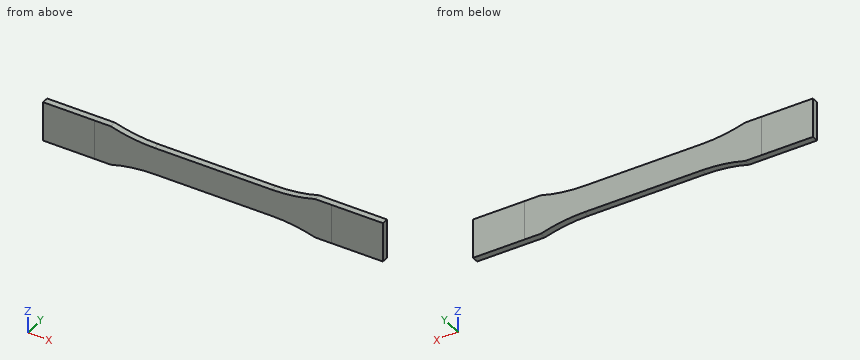
```python
from build123d import *

# Parameters (mm, degrees)
CROQUIS1_W              = 57
CROQUIS1_H              = 13
SALIENTE_EXTRUIR1_DEPTH = 1.6
CROQUIS2_W              = 25
CROQUIS2_H              = 19
CORTAR_EXTRUIR1_DEPTH   = 0.01


with BuildPart() as part:
    # Croquis1 → Saliente-Extruir1 (new body, symmetric)
    with BuildSketch(Plane(origin=(0, 0, 0), x_dir=(1, 0, 0), z_dir=(0, 1, 0))):
        with BuildLine():
            Line((-82.5, -9.5), (-49.642374512, -9.5))
            ThreePointArc((-49.642374512, -9.5), (-39.177078252, -7.253737634), (-28.5, -6.5))
            Line((-28.5, -6.5), (-28.5, 6.5))
            ThreePointArc((-28.5, 6.5), (-39.177078252, 7.253737634), (-49.642374512, 9.5))
            Line((-49.642374512, 9.5), (-82.5, 9.5))
            Line((-82.5, 9.5), (-82.5, -9.5))
        make_face()
        with BuildLine():
            Line((49.642374512, -9.5), (82.5, -9.5))
            Line((82.5, -9.5), (82.5, 9.5))
            Line((82.5, 9.5), (49.642374512, 9.5))
            ThreePointArc((49.642374512, 9.5), (39.177078252, 7.253737634), (28.5, 6.5))
            Line((28.5, 6.5), (28.5, -6.5))
            ThreePointArc((28.5, -6.5), (39.177078252, -7.253737634), (49.642374512, -9.5))
        make_face()
        Rectangle(CROQUIS1_W, CROQUIS1_H)
    extrude(amount=SALIENTE_EXTRUIR1_DEPTH, both=True)

    # Croquis2 → Cortar-Extruir1 (cut)
    with BuildSketch(Plane(origin=(0, 1.6, 0), x_dir=(1, 0, 0), z_dir=(0, 1, 0))):
        with Locations((-70, 0)):
            Rectangle(CROQUIS2_W, CROQUIS2_H)
        with Locations((70, 0)):
            Rectangle(CROQUIS2_W, CROQUIS2_H)
    cortar_extruir1 = extrude(amount=-CORTAR_EXTRUIR1_DEPTH, mode=Mode.SUBTRACT)

    # Simetría1: Cortar-Extruir1 across plane
    add(cortar_extruir1.mirror(Plane.ZX), mode=Mode.SUBTRACT)


solid = part.part
```
Source: CAD feature listing. Evaluate the final solid. Frame: model axes, mm. Round coordinates to 2 decimals unless told otherwise and drop trailing zeros. Loops run counter-clockwise (first coordinate to the right, second up) from the corner with the lowest first, then second, coordinate; pieces in that order, holes last.
1. Section query A-A on y = 0.75. Output: boundary loops of the cut face in (x, z), and give its area (3 significant figures).
2. Section query B-B on x = -1. Output: boundary loops of the cut face in (y, z), and give its area (3 significant figures).
3. Ray query, L1, parallel to Y at x = -69.5, z = 2.5; L2, parallel to Z at x = -2, y = -0.75; L3, parallel to Z at x = 36, y = -1. Return the intervals inside material, ascending.
4. Contact query for flat-ended pins moving along their axis: pin 1 (5.5 mm diameter, centred on x = 73.5, z = 2, fed in from -Y); pin 2 (5.5 mm diameter, centred on x = 72, z = 1, fed in from +Y); pin 3 (1.6 mm diameter, centred on x = -3, y = -0.5, fed in from +Z). Output: stop coordinate, or through.
5. Section query C-C on x = -44. Output: boundary loops of the cut face in (y, z).
Answers below:
1. outline: (-82.5, -9.5) - (-49.64, -9.5) arc R76 cw to (-28.5, -6.5) - (28.5, -6.5) arc R76 cw to (49.64, -9.5) - (82.5, -9.5) - (82.5, 9.5) - (49.64, 9.5) arc R76 cw to (28.5, 6.5) - (-28.5, 6.5) arc R76 cw to (-49.64, 9.5) - (-82.5, 9.5) - close
1. area: 2,620 mm2
2. outline: (-1.6, -6.5) - (1.6, -6.5) - (1.6, 6.5) - (-1.6, 6.5) - close
2. area: 41.6 mm2
3. L1: y = -1.59 to 1.59
3. L2: z = -6.5 to 6.5
3. L3: z = -6.87 to 6.87
4. pin 1: stops at y = -1.59
4. pin 2: stops at y = 1.59
4. pin 3: stops at z = 6.5
5. outline: (-1.6, -8.1) - (1.6, -8.1) - (1.6, 8.1) - (-1.6, 8.1) - close
